Autodesk Inventor part; units mm, degrees
ref_plane "YZ Plane" through (0, 0, 0) normal (1, 0, 0) x (0, 1, 0)
ref_plane "XZ Plane" through (0, 0, 0) normal (0, 1, 0) x (-1, 0, 0)
ref_plane "XY Plane" through (0, 0, 0) normal (0, 0, 1) x (1, 0, 0)
sketch "Sketch1" plane through (0, 0, 0) normal (0, 1, 0) x (-1, 0, 0)
  circle A0 centre (0, 0) radius 20
  circle A1 centre (0, 0) radius 11
  circle A2 centre (0, 0) radius 5
  dimension "d0" = 40
  dimension "d1" = 22
  dimension "d4" = 10
extrude "Extrusion1" add sketch "Sketch1" along normal blind 7 contours A0 | A1 | A2
extrude "Extrusion2" add sketch "Sketch1" against normal blind 20 contours A1
properties part number "11T-Sprocket"
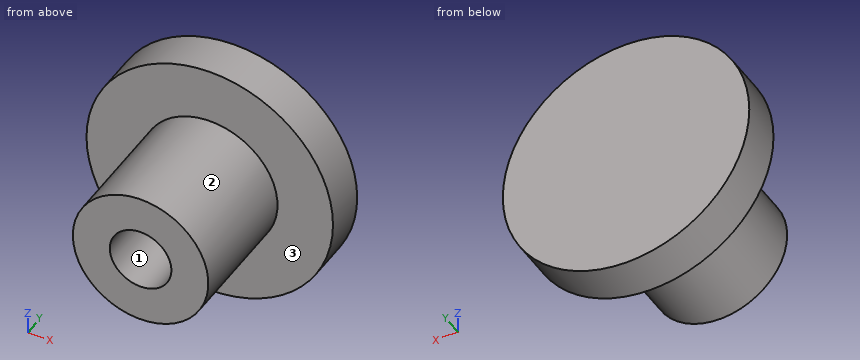
Read the model definition and answer for the solid it produces. Units are mm, in the model's axes. Face numbers are marked on the shaded views. Coordinates: 2 decimals unless noted, no trailing zeros. Order: outer loops, then holes, each group sorted by start corner. A loop starts at its lowest first (then second) coordinate and runs counter-clockwise, first axis right, second up. Notation, with made-up numbers: M -6,60.25 L 39,60.25 A23 ccw 39,97.25 Z; hole C 13,-30.5 d10. An arc over 180 degrees is marked long. Put each result on its own line as item: value. Start each with the question number.
Item 1: Section C-C, the plane y = -9.5 is taken. Determine the outline of the cut face in (x, z).
Item 2: Section A-A, the plane x = 0 is taken. Determine the outline of the cut face in (y, z), plus the area to 3 significant figures.
Item 3: Consider probe 1 along Z at (x, y) = (0, -9.5); probe 2 along Y at (x, z) = (13, -13); probe 3 along X at (y, z) = (-10.25, -2). Determine where each line is inside the solid, lowest interval first. Write a range as [from, to].
Item 4: The mould has two halves that part along Z. Classify the marked faces 1, 2 and 3: +Z half, -Z half, draft (parallel to the pull), parting line (faces both ways), or undercut.
Item 5: Given pin 1 Ø2 at (y, z) = (-3, 0) entering from -X; pin 2 Ø4 at (y, z) = (-9, -10) entering from -X; pin 3 Ø5 at (x, z) = (-1.5, -1) entering from -Y, each flat-ended and moving along its own axis, determine where each tip first touches the part or whether it passes through.
Item 6: Section B-B, the plane z = 0 is taken. Determine the outline of the cut face in (x, y), plus the area to 3 significant figures.
Item 7: Section D-D, the plane z = 8 is taken. Determine the outline of the cut face in (x, y).
Computed:
1. outline: C 0,0 d22; hole C 0,0 d10
2. outline: M -20,-11 L 0,-11 L 0,-20 L 7,-20 L 7,20 L 0,20 L 0,11 L -20,11 L -20,5 L 0,5 L 0,-5 L -20,-5 Z
2. area: 520 mm2
3. probe 1: z = [-11, -5], [5, 11]
3. probe 2: y = [0, 7]
3. probe 3: x = [-10.82, -4.58], [4.58, 10.82]
4. face 1: undercut
4. face 2: parting line
4. face 3: draft
5. pin 1: stops at x = -11
5. pin 2: stops at x = -7.55
5. pin 3: stops at y = 0
6. outline: M -20,0 L -11,0 L -11,-20 L -5,-20 L -5,0 L 5,0 L 5,-20 L 11,-20 L 11,0 L 20,0 L 20,7 L -20,7 Z
6. area: 520 mm2
7. outline: M -18.33,0 L -7.55,0 L -7.55,-20 L 7.55,-20 L 7.55,0 L 18.33,0 L 18.33,7 L -18.33,7 Z
